```python
from build123d import *

# Parameters (mm, degrees)
SKETCH_2_R      = 2.35
EXTRUDE_2_DEPTH = 5
SKETCH_3_R      = 4
EXTRUDE_4_DEPTH = 5


with BuildPart() as part:
    # Эскиз2 → Бобышка-Вытянуть2 (new body)
    with BuildSketch(Plane.XY.offset(31.602998)):
        Circle(SKETCH_2_R)
        with BuildLine():
            Line((0, 3.25), (-0.83598392, 2.196276596))
            ThreePointArc((-0.83598392, 2.196276596), (0, 2.35), (0.83598392, 2.196276596))
            Line((0.83598392, 2.196276596), (0, 3.25))
        make_face()
        with BuildLine():
            Line((2.814582562, 1.625), (1.484039366, 1.82212161))
            ThreePointArc((1.484039366, 1.82212161), (2.035159699, 1.175), (2.320023286, 0.374154986))
            Line((2.320023286, 0.374154986), (2.814582562, 1.625))
        make_face()
        with BuildLine():
            Line((2.814582562, -1.625), (2.320023286, -0.374154986))
            ThreePointArc((2.320023286, -0.374154986), (2.035159699, -1.175), (1.484039366, -1.82212161))
            Line((1.484039366, -1.82212161), (2.814582562, -1.625))
        make_face()
        with BuildLine():
            ThreePointArc((0.83598392, -2.196276596), (0, -2.35), (-0.83598392, -2.196276596))
            Line((-0.83598392, -2.196276596), (0, -3.25))
            Line((0, -3.25), (0.83598392, -2.196276596))
        make_face()
        with BuildLine():
            ThreePointArc((-1.484039366, -1.82212161), (-2.035159699, -1.175), (-2.320023286, -0.374154986))
            Line((-2.320023286, -0.374154986), (-2.814582562, -1.625))
            Line((-2.814582562, -1.625), (-1.484039366, -1.82212161))
        make_face()
        with BuildLine():
            ThreePointArc((-2.320023286, 0.374154986), (-2.035159699, 1.175), (-1.484039366, 1.82212161))
            Line((-1.484039366, 1.82212161), (-2.814582562, 1.625))
            Line((-2.814582562, 1.625), (-2.320023286, 0.374154986))
        make_face()
    extrude(amount=EXTRUDE_2_DEPTH)

    # Эскиз3 → Бобышка-Вытянуть4 (add)
    with BuildSketch(Plane.XY.offset(31.602998)):
        Circle(SKETCH_3_R)
    extrude(amount=-EXTRUDE_4_DEPTH)


solid = part.part
```
Geometry check sheet. Reference: the model listing, model coordinates, mm. A direction names the side the tool comes from. Coordinates: 2 decimals unless noted, no trailing zeros. Write each loop counter-clockwise with the first axis right and the second up, starting at its lowest first coordinate (ties: lowest second). Pieces come first, ordered by that corner, then holes. Notation, with made-up numbers: M 63.25,85.5 L 105.25,85.5 A30 cw 105.25,112.5 Z; hole C 20.25,-25.75 d1. An arc over 180 degrees is marked long. One line per item, written item: value. Start each with the question number.
(1) Sectioned sample at D-D, the plane x = -2.5. Enter the section's corners in (y, z), and give its area (3 significant figures).
(2) Release check for a two-part mould opening along Y. For faces 1 (the face through (-0.41, 2.73, 34.07)), 2 (the face through (0.41, -2.73, 34.07)), 3 (the face through (-2.57, 1.01, 34.07)), 4 (the face through (2.57, -1.01, 34.07)) record: released by +Y, released by -Y, zero draft, split by the parting line, or undercut.
(3) Tool access check on faces 5 (the face through (-2.564, -0.991, 34.068)), 6 (the face through (2.16, 1.72, 34.07)), 7 (the face through (2, 2, 31.603)). Record the directions out of +Z, -Z, +X, -X, +Y, -Y that give a thin tool (end or side, any length) a straight path to the whole face; none if there is none.
(4) Depth check by flat-ended pin: pin 1 (1 mm diameter, centred on y = -2, z = 34, fed in from -X); pin 2 (2 mm diameter, centred on x = -1.5, z = 29, fed in from +Y). Enter the tip coordinate at first touch or a pass-through.
(5) Sectioned sample at B-B, the plane z = 32.75. Enter the section's corners in (x, y) (3 decimals).
(6) Scan lines: line 1 along Z through (x, y) = (-3, 1.25); line 2 along Y through (x, z) = (-1.5, 35.75); line 3 along X through (y, z) = (0, 34). Record each from-to range of solid material in increasing order. Write a range as [from, to].
(7) Sectioned sample at C-C, the plane x = 1.25. Enter the section's corners in (y, z).
(8) Sectioned sample at A-A, the plane y = 0. Enter the section's corners in (x, z).
Filled sheet:
1. outline: M -3.12,26.6 L 3.12,26.6 L 3.12,31.6 L 1.67,31.6 L 1.67,36.6 L 0.83,36.6 L 0.83,31.6 L -0.83,31.6 L -0.83,36.6 L -1.67,36.6 L -1.67,31.6 L -3.12,31.6 Z
1. area: 39.6 mm²
2. face 1: released by +Y
2. face 2: released by -Y
2. face 3: undercut
2. face 4: undercut
3. face 5: +Z, -X
3. face 6: +Z, +X, +Y
3. face 7: +Z
4. pin 1: x = -2.81
4. pin 2: y = 3.97
5. outline: M -2.815,-1.625 L -1.484,-1.822 A2.35 ccw -0.836,-2.196 L 0,-3.25 L 0.836,-2.196 A2.35 ccw 1.484,-1.822 L 2.815,-1.625 L 2.32,-0.374 A2.35 ccw 2.32,0.374 L 2.815,1.625 L 1.484,1.822 A2.35 ccw 0.836,2.196 L 0,3.25 L -0.836,2.196 A2.35 ccw -1.484,1.822 L -2.815,1.625 L -2.32,0.374 A2.35 ccw -2.32,-0.374 Z
6. line 1: [26.6, 31.6]
6. line 2: [-1.82, 1.82]
6. line 3: [-2.35, 2.35]
7. outline: M -3.8,26.6 L 3.8,26.6 L 3.8,31.6 L 1.99,31.6 L 1.99,36.6 L -1.99,36.6 L -1.99,31.6 L -3.8,31.6 Z
8. outline: M -4,26.6 L 4,26.6 L 4,31.6 L 2.35,31.6 L 2.35,36.6 L -2.35,36.6 L -2.35,31.6 L -4,31.6 Z
